from build123d import *

# Parameters (mm, degrees)
BOSS_EXTRUDE2_DEPTH = 5
BOSS_EXTRUDE3_DEPTH = 2.9
CUT_EXTRUDE1_REACH  = 24.353
SKETCH5_R           = 2.6


with BuildPart() as part:
    # Sketch3 → Boss-Extrude2 (new, symmetric)
    with BuildSketch(Plane.XY):
        with BuildLine():
            Line((0, -15), (0, 15))
            Line((0, 15), (11.8, 15))
            Line((11.8, 15), (11.8, 7.795511529))
            ThreePointArc((11.8, 7.795511529), (6.150961765, -2.000649589), (15.8, -7.897467949))
            Line((15.8, -7.897467949), (15.8, -15))
            Line((15.8, -15), (0, -15))
        make_face()
    extrude(amount=BOSS_EXTRUDE2_DEPTH, both=True)

    # Sketch4 → Boss-Extrude3 (add, symmetric)
    with BuildSketch(Plane.XY):
        with BuildLine():
            Line((11.8, 8.21035931), (11.8, 5.582114295))
            ThreePointArc((11.8, 5.582114295), (8.343588332, -2.001251369), (15.8, -5.723635209))
            Line((15.8, -5.723635209), (15.8, -8.30722577))
            ThreePointArc((15.8, -8.30722577), (5.738786153, -2.000586358), (11.8, 8.21035931))
        make_face()
    extrude(amount=BOSS_EXTRUDE3_DEPTH, both=True)

    # Sketch5 → Cut-Extrude1 (cut, up to next)
    with BuildSketch(Plane(origin=(0, 0, 0), x_dir=(0, 0, -1), z_dir=(1, 0, 0)), mode=Mode.PRIVATE) as cut_extrude1_sk1:
        with Locations(Location((0, 11, 0), (0, 0, 270))):
            Circle(SKETCH5_R)
    cut_extrude1_tool1 = extrude(cut_extrude1_sk1.sketch, amount=CUT_EXTRUDE1_REACH, mode=Mode.PRIVATE) & part.part
    # Sketch5 → Cut-Extrude1 (cut, up to next)
    with BuildSketch(Plane(origin=(0, 0, 0), x_dir=(0, 0, -1), z_dir=(1, 0, 0)), mode=Mode.PRIVATE) as cut_extrude1_sk2:
        with Locations(Location((0, -11, 0), (0, 0, 180))):
            Circle(SKETCH5_R)
    cut_extrude1_tool2 = extrude(cut_extrude1_sk2.sketch, amount=CUT_EXTRUDE1_REACH, mode=Mode.PRIVATE) & part.part
    add(cut_extrude1_tool1.solids().sort_by_distance((0, 11, 0))[0], mode=Mode.SUBTRACT)
    add(cut_extrude1_tool2.solids().sort_by_distance((0, -11, 0))[0], mode=Mode.SUBTRACT)


solid = part.part
Geometry: final body of the model. Coordinates: model frame, mm. A direction names the side the tool comes from. Coordinates: 2 decimals unless noted, no trailing zeros. Loops run counter-clockwise (first coordinate to the right, second up) from the corner with the lowest first, then second, coordinate; pieces in that order, holes last. Notation, with made-up numbers: M 12,45.25 L 16,45.25 A35 cw 16,83.25 Z; hole C 55,87 d11. An arc over 180 degrees is marked long. One line per item, written item: value. Start each with the question number.
1) Material intervals for L1, parallel to Z at x = 4, y = -11; L2, parallel to Y at x = 4, z = -1.5; L3, parallel to Y at x = 10.25, z = 2, sorted ascending. Write a range as from..to.
2) Cut plane A-A (y = -11). Return loops of the section in (x, z), then the cut area to 3 significant figures.
3) Pin query (flat end, axial travel): P1, Ø5, axis at y = -5.5, z = 2.5, coming from the -X side; P2, Ø4.5, axis at y = 10, z = 2, coming from the +X side; P3, Ø5, axis at x = 9, y = 2, coming from the -Z side; P4, Ø2, axis at y = -1, z = 2.5, coming from the +X side. Return the tip coordinate at first contact, or that it passes through.
4) Cut plane B-B (z = 0). Return loops of the section in (x, y).
5) Draft query along Y for faces 1 (the cylindrical face through (8.302, -1.879, 0.041)), 2 (the flat face through (0, 0, 0)), 3 (the flat face through (6, 15, 0)). Return one class per face: released by +Y, released by -Y, zero draft, split by the parting line, or undercut.
6) Reachability of faces 4 (the flat face through (8, -15, 0)), 5 (the flat face through (11.8, 8, 0)) from +Z, -Z, +X, -X, +Y, -Y: full face, straight path, thin tool, end or side. Return the list, or none.
7) Cut plane C-C (x = 11). Return loops of the section in (y, z).
8) Cut plane D-D (x = 14). Return loops of the section in (y, z).
Evaluation:
1. L1: -5..-2.6, 2.6..5
1. L2: -15..-13.12, -8.88..8.88, 13.12..15
1. L3: -15..-12.66, -9.34..-4.68, 4.68..9.34, 12.66..15
2. outline: M 0,-5 L 15.8,-5 L 15.8,-2.6 L 0,-2.6 Z; M 0,2.6 L 15.8,2.6 L 15.8,5 L 0,5 Z
2. area: 75.8 mm^2
3. P1: x = 0
3. P2: x = 11.8
3. P3: z = -2.9
3. P4: x = 8.34
4. outline: M 0,-15 L 15.8,-15 L 15.8,-13.6 L 0,-13.6 Z; M 0,-8.4 L 15.8,-8.4 L 15.8,-5.72 A6 cw 11.8,5.58 L 11.8,8.4 L 0,8.4 Z; M 0,13.6 L 11.8,13.6 L 11.8,15 L 0,15 Z
5. face 1: undercut
5. face 2: zero draft
5. face 3: released by +Y
6. face 4: +Z, -Z, +X, -X, -Y
6. face 5: +Z, -Z, +X, +Y
7. outline: M -15,-5 L -7.52,-5 L -7.52,-2.9 L -5.2,-2.9 L -5.2,2.9 L -7.52,2.9 L -7.52,5 L -15,5 Z; M 5.2,-2.9 L 7.52,-2.9 L 7.52,-5 L 15,-5 L 15,5 L 7.52,5 L 7.52,2.9 L 5.2,2.9 Z; hole C -11,0 d5.2; hole C 11,0 d5.2
8. outline: M -15,-5 L -8.1,-5 L -8.1,-2.9 L -6,-2.9 L -6,2.9 L -8.1,2.9 L -8.1,5 L -15,5 Z; hole C -11,0 d5.2
